Part model, mm, in its own coordinate system. Face numbers are marked on the shaded views. A direction names the side the tool comes from. Give positions to 0.01 mm unless a question says otherwise; leave off trailing zeros. Loops run counter-clockwise (first coordinate to the right, second up) from the corner with the lowest first, then second, coordinate; pieces in that order, holes last. Notation, with made-up numbers: M 67.25,11 L 94.25,11 A19 cw 94.25,43 Z; hole C 76.5,11 d3. An arc over 180 degrees is marked long. Answer in a Markdown table with one row per item.
from build123d import *

# Parameters (mm, degrees)
F1_DEPTH = 69.85
F2_W     = 101.6
F2_H     = 34.268197
F3_DEPTH = 15.875
F4_W     = 22.225
F4_H     = 69.85
F5_DEPTH = 22.225


with BuildPart() as f1:
    # F0 (on Top) → F1 (new body)
    with BuildSketch(Plane.XY):
        Polygon((67.618918, 15.875), (-72.081082, 15.875), (-72.081082, 0), (23.168918, 0), (29.518918, 0), (29.518918, 6.35), (51.743918, 6.35), (67.618918, 6.35), align=None)
    extrude(amount=-F1_DEPTH)

    # F2 (on Front) → F3 (join)
    with BuildSketch(Plane.XZ):
        with Locations((-21.070717, -52.628895)):
            Rectangle(F2_W, F2_H)
    extrude(amount=F3_DEPTH)

    # F4 (on face) → F5 (join)
    with BuildSketch(Plane.XZ.offset(-6.35)):
        with Locations((40.631418, -34.925)):
            Rectangle(F4_W, F4_H)
    extrude(amount=F5_DEPTH)


solid = f1.part
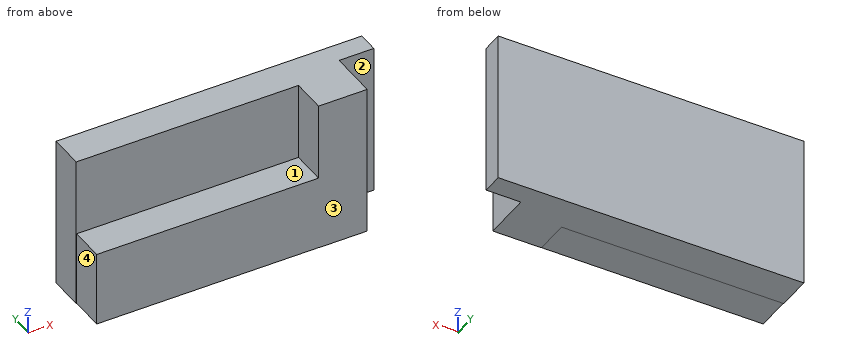
(1) Saw through at B-B (x = 20.5). Write the cut outline in (y, z) (3 decimals), plus the area to 3 significant figures.
Recorded:
| item | result |
|---|---|
| outline | M -15.875,-69.763 L 0,-69.763 L 0,-69.85 L 15.875,-69.85 L 15.875,0 L 0,0 L 0,-35.495 L -15.875,-35.495 Z |
| area | 1,650 mm^2 |
(2) Pin check, flat tips, straight feed: pin 1 Ø2 at (x, z) = (-46, -29) entering from -Y; pin 2 Ø5 at (x, y) = (-30.5, -10) entering from -Z; pin 3 Ø4 at (y, z) = (-5, -27.5) entering from +X. Stop position of each tip, or through.
Recorded:
| item | result |
|---|---|
| pin 1 | stops at y = 0 |
| pin 2 | stops at z = -69.76 |
| pin 3 | stops at x = 51.74 |
(3) Saw through at D-D (x = 54.5). Write the cut outline in (y, z) (3 decimals), plus the area to 3 significant figures.
Recorded:
| item | result |
|---|---|
| outline | M 6.35,-69.85 L 15.875,-69.85 L 15.875,0 L 6.35,0 Z |
| area | 665 mm^2 |
(4) Drill centre lines: line 1 along Y through (x, z) = (26, -13.5) (3 decimals); line 2 along Z through (x, y) = (7, -9); line 3 along X through (y, z) = (-12, -62.5). Where is each one in solid material? Low to high.
Recorded:
| item | result |
|---|---|
| line 1 | y = 0 to 15.875 |
| line 2 | z = -69.76 to -35.49 |
| line 3 | x = -71.87 to 51.74 |
(5) Saw through at A-A (z = -21). Write the cut outline in (x, y) (3 decimals), plus the area to 3 significant figures.
Recorded:
| item | result |
|---|---|
| outline | M -72.081,0 L 29.519,0 L 29.519,-15.875 L 51.744,-15.875 L 51.744,6.35 L 67.619,6.35 L 67.619,15.875 L -72.081,15.875 Z |
| area | 2,470 mm^2 |
(6) Which spindle directions (+Z, -Z, +X, -X, +Y, -Y) get a long thin tool onto all of the face, cutting with end or side? Do the marked faces 1, 2, 3 and 4. Say none if no direction does.
Recorded:
| item | result |
|---|---|
| face 1 | +Z, -X, -Y |
| face 2 | +Z, -Z, +X, -Y |
| face 3 | +Z, -Z, +X, -X, -Y |
| face 4 | +Z, -Z, -X, -Y |
(7) Saw through at C-C (y = 3). Write the cut outline in (x, z).
Recorded:
| item | result |
|---|---|
| outline | M -72.08,-69.85 L 51.74,-69.85 L 51.74,0 L -72.08,0 Z |
